Here's how the part is built. I have some questions about the finished solid (model axes, mm). Face numbers are marked on the shaded views. A direction names the side the tool comes from. Coordinates: 2 decimals unless noted, no trailing zeros. Loops run counter-clockwise (first coordinate to the right, second up) from the corner with the lowest first, then second, coordinate; pieces in that order, holes last. Notation, with made-up numbers: M 34,29.25 L 52,29.25 A28 ccw 52,56.25 Z; hole C 47,73.25 d8. An arc over 180 degrees is marked long. Use one line per item in the form item = value. Start each with the question number.
(1) Will these pins go through, and if not, where does the flat tip stop? P1, Ø6, axis at x = 93, y = 13, coming from the -Z side; P2, Ø6, axis at y = 26, z = -1.5, coming from the +X side; P3, Ø1.6, axis at x = -0.5, y = 3, coming from the +Z side.
(2) Thinking about a two-plate mould opening in X: for the marked faces 1 and 2, which applies, +X half, -X half, draft (parallel to the pull), parting line (faces both ways), or undercut?
(3) Please list where these lines run through material, in increasing order: L1, parallel to X at y = 30, z = -6.5; L2, parallel to Y at x = 18.15, z = 0; L3, parallel to Y at x = 23, z = 13.
(4) Imagine slicing it at C-C, the plane y = 18.5. Please give me the cut outline in (x, z).
(5) Imagine slicing it at B-B, the plane x = 23.5. Please give me the cut outline in (y, z).
(6) On a 3-axis mill with a long thin cutter (end or side, diameter ignored), from which of +Z, -Z, +X, -X, +Y, -Y can I reach the whole of each face in a straight line? I mean the marked faces 3 and 4. Say none if no direction works.
(7) Imagine slicing it at A-A, the plane y = 7. Please give me the cut outline in (x, z).
(8) Imagine slicing it at D-D, the plane z = -12.5. Please give me the cut outline in (x, y), and give its area (3 significant figures).
```python
from build123d import *

# Parameters (mm, degrees)
EXTRUDE_1_DEPTH     = 2
SKETCH_2_W          = 90
SKETCH_2_H          = 20
EXTRUDE_2_DEPTH     = 3
SKETCH_3_W          = 10
SKETCH_3_H          = 20
SKETCH_3_W_2        = 5.5
SKETCH_3_W_3        = 7
EXTRUDE_3_DEPTH     = 30
SKETCH_4_R          = 3.25
CUT_EXTRUDE_1_DEPTH = 4
SKETCH_5_W          = 13.678161833
SKETCH_5_H          = 1.5
SKETCH_5_W_2        = 1.5
SKETCH_5_H_2        = 16.732170562
SKETCH_5_H_3        = 11.514895911
EXTRUDE_4_DEPTH     = 4


with BuildPart() as part:
    # 草图1 → 凸台-拉伸1 (new body)
    with BuildSketch(Plane(origin=(0, 0, 0), x_dir=(1, 0, 0), z_dir=(0, 1, 0))):
        Polygon((10, 15), (10, 10), (0, 10), (0, -10), (10, -10), (10, -15), (110, -15), (110, 15), align=None)
    extrude(amount=EXTRUDE_1_DEPTH)

    # 草图2 → 凸台-拉伸2 (add)
    with BuildSketch(Plane(origin=(0, 2, 0), x_dir=(1, 0, 0), z_dir=(0, 1, 0))):
        with Locations((60, 0)):
            Rectangle(SKETCH_2_W, SKETCH_2_H)
    extrude(amount=EXTRUDE_2_DEPTH)

    # 草图3 → 凸台-拉伸3 (add)
    with BuildSketch(Plane(origin=(0, 5, 0), x_dir=(1, 0, 0), z_dir=(0, 1, 0))):
        with Locations((85.5, 0)):
            Rectangle(SKETCH_3_W, SKETCH_3_H)
        with Locations((68, 0)):
            Rectangle(SKETCH_3_W, SKETCH_3_H)
        with Locations((50.5, 0)):
            Rectangle(SKETCH_3_W, SKETCH_3_H)
        with Locations((33, 0)):
            Rectangle(SKETCH_3_W, SKETCH_3_H)
        with Locations((17.75, 0)):
            Rectangle(SKETCH_3_W_2, SKETCH_3_H)
        with Locations((101.5, 0)):
            Rectangle(SKETCH_3_W_3, SKETCH_3_H)
    extrude(amount=EXTRUDE_3_DEPTH)

    # 草图4 → 切除-拉伸1 (cut)
    with BuildSketch(Plane.ZY.offset(-15)):
        with Locations((0, 7)):
            Circle(SKETCH_4_R)
    extrude(amount=-CUT_EXTRUDE_1_DEPTH, mode=Mode.SUBTRACT)

    # 草图5 → 凸台-拉伸4 (add)
    with BuildSketch(Plane(origin=(0, 0, 0), x_dir=(1, 0, 0), z_dir=(0, 1, 0))):
        with Locations((58.012206535, -15.75)):
            Rectangle(SKETCH_5_W, SKETCH_5_H)
        with Locations((58.012206535, 15.75)):
            Rectangle(SKETCH_5_W, SKETCH_5_H)
        with Locations((110.75, -0.281087738)):
            Rectangle(SKETCH_5_W_2, SKETCH_5_H_2)
        with Locations((-0.75, -0.048934151)):
            Rectangle(SKETCH_5_W_2, SKETCH_5_H_3)
    extrude(amount=EXTRUDE_4_DEPTH)


solid = part.part
```
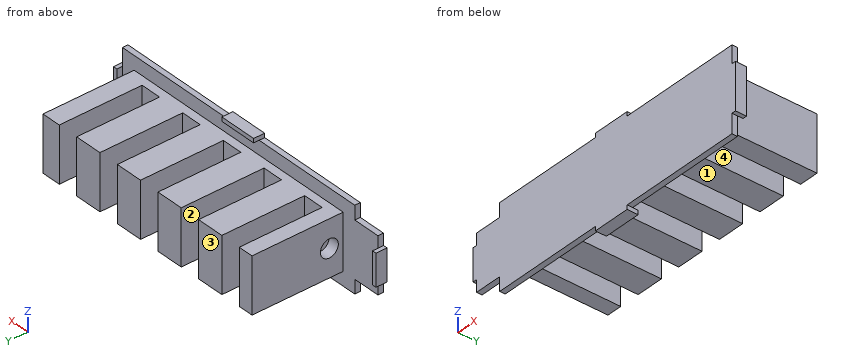
Answer:
q1.P1 = -10
q1.P2 = 105
q1.P3 = 5.81
q2.face_1 = draft
q2.face_2 = undercut
q3.L1 = 15 to 20.5, 28 to 38, 45.5 to 55.5, 63 to 73, 80.5 to 90.5, 98 to 105
q3.L2 = 0 to 3.75, 10.25 to 35
q3.L3 = 0 to 2
q4.outline = M 15,-10 L 20.5,-10 L 20.5,10 L 15,10 Z; M 28,-10 L 38,-10 L 38,10 L 28,10 Z; M 45.5,-10 L 55.5,-10 L 55.5,10 L 45.5,10 Z; M 63,-10 L 73,-10 L 73,10 L 63,10 Z; M 80.5,-10 L 90.5,-10 L 90.5,10 L 80.5,10 Z; M 98,-10 L 105,-10 L 105,10 L 98,10 Z
q5.outline = M 0,-15 L 2,-15 L 2,-10 L 5,-10 L 5,10 L 2,10 L 2,15 L 0,15 Z
q6.face_3 = +Z, -Z, +X, -X, +Y
q6.face_4 = +Z, -Z, +Y
q7.outline = M 15,-10 L 20.5,-10 L 20.5,10 L 15,10 L 15,3.25 L 19,3.25 L 19,-3.25 L 15,-3.25 Z; M 28,-10 L 38,-10 L 38,10 L 28,10 Z; M 45.5,-10 L 55.5,-10 L 55.5,10 L 45.5,10 Z; M 63,-10 L 73,-10 L 73,10 L 63,10 Z; M 80.5,-10 L 90.5,-10 L 90.5,10 L 80.5,10 Z; M 98,-10 L 105,-10 L 105,10 L 98,10 Z
q8.outline = M 10,0 L 110,0 L 110,2 L 10,2 Z
q8.area = 200 mm²
